Geometry check sheet. Reference: the model listing, model coordinates, mm. Face numbers are marked on the shaded views. Give positions to 0.01 mm unless a question says otherwise; leave off trailing zeros. Loops run counter-clockwise (first coordinate to the right, second up) from the corner with the lowest first, then second, coordinate; pieces in that order, holes last. Notation, with made-up numbers: (44, 46.25) -> (49, 46.25) arc R24 ccw to (49, 65.25) -> close; hole circle Ø11 at (5.25, 17.25). An arc over 180 degrees is marked (long way). Answer as a JSON object with one key per item and string values.
from build123d import *

# Parameters (mm, degrees)
CROQUIS1_W              = 60
CROQUIS1_H              = 116
CROQUIS1_R              = 1.5
SALIENTE_EXTRUIR1_DEPTH = 15
CROQUIS2_W              = 15
CROQUIS2_H              = 15
CORTAR_EXTRUIR1_DEPTH   = 132.457217375


with BuildPart() as part:
    # Croquis1 → Saliente-Extruir1 (new body)
    with BuildSketch(Plane(origin=(0, 0, 0), x_dir=(0, 0, -1), z_dir=(1, 0, 0))):
        with Locations((30, 58)):
            Rectangle(CROQUIS1_W, CROQUIS1_H)
        with Locations((54, 5)):
            Circle(CROQUIS1_R, mode=Mode.SUBTRACT)
        with Locations((36, 5)):
            Circle(CROQUIS1_R, mode=Mode.SUBTRACT)
        with Locations((36, 29)):
            Circle(CROQUIS1_R, mode=Mode.SUBTRACT)
        with Locations((54, 29)):
            Circle(CROQUIS1_R, mode=Mode.SUBTRACT)
        with Locations(Location((24, 29, 0), (0, 0, 180))):
            Circle(CROQUIS1_R, mode=Mode.SUBTRACT)
        with Locations(Location((24, 5, 0), (0, 0, 180))):
            Circle(CROQUIS1_R, mode=Mode.SUBTRACT)
        with Locations(Location((6, 5, 0), (0, 0, 180))):
            Circle(CROQUIS1_R, mode=Mode.SUBTRACT)
        with Locations(Location((6, 29, 0), (0, 0, 180))):
            Circle(CROQUIS1_R, mode=Mode.SUBTRACT)
        with Locations((6, 87)):
            Circle(CROQUIS1_R, mode=Mode.SUBTRACT)
        with Locations((6, 111)):
            Circle(CROQUIS1_R, mode=Mode.SUBTRACT)
        with Locations((24, 111)):
            Circle(CROQUIS1_R, mode=Mode.SUBTRACT)
        with Locations((24, 87)):
            Circle(CROQUIS1_R, mode=Mode.SUBTRACT)
        with Locations(Location((36, 87, 0), (0, 0, 180))):
            Circle(CROQUIS1_R, mode=Mode.SUBTRACT)
        with Locations(Location((36, 111, 0), (0, 0, 180))):
            Circle(CROQUIS1_R, mode=Mode.SUBTRACT)
        with Locations(Location((54, 111, 0), (0, 0, 180))):
            Circle(CROQUIS1_R, mode=Mode.SUBTRACT)
        with Locations(Location((54, 87, 0), (0, 0, 180))):
            Circle(CROQUIS1_R, mode=Mode.SUBTRACT)
        with Locations((32.5, 76.8)):
            Circle(CROQUIS1_R, mode=Mode.SUBTRACT)
        with Locations((32.5, 39.2)):
            Circle(CROQUIS1_R, mode=Mode.SUBTRACT)
    extrude(amount=SALIENTE_EXTRUIR1_DEPTH)

    # Croquis2 → Cortar-Extruir1 (cut, through all)
    with BuildSketch(Plane(origin=(15, 0, 0), x_dir=(0, 0, -1), z_dir=(1, 0, 0))):
        with Locations((7.5, 65.5)):
            Rectangle(CROQUIS2_W, CROQUIS2_H)
        with Locations((52.5, 50.5)):
            Rectangle(CROQUIS2_W, CROQUIS2_H)
    extrude(amount=-CORTAR_EXTRUIR1_DEPTH, mode=Mode.SUBTRACT)


solid = part.part
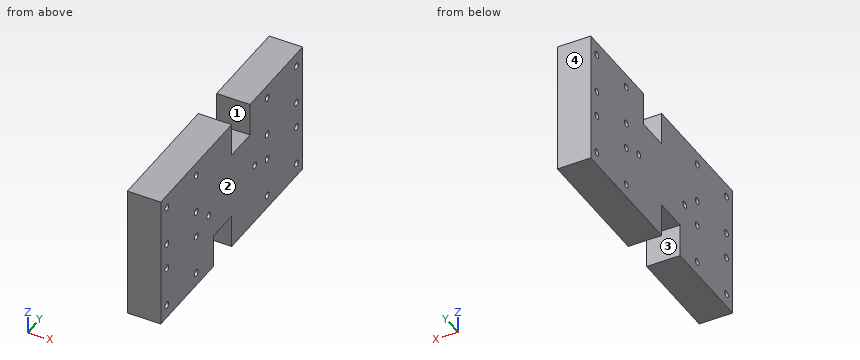
1) Section check A-A on z = -12. Record the cut outline in (x, y).
Geometry check:
{"outline": "(0, 0) -> (15, 0) -> (15, 58) -> (0, 58) -> close; (0, 73) -> (15, 73) -> (15, 116) -> (0, 116) -> close"}
2) Material ranges on line 1 along Z through (x, y) = (7.5, 111); line 2 along Y through (x, z) = (10, -36); line 3 along Y through (x, z) = (10.75, -6), recorded low to high. Write a range as from..to.
Geometry check:
{"line 1": "z = -60..-55.5, -52.5..-37.5, -34.5..-25.5, -22.5..-7.5, -4.5..0", "line 2": "y = 0..3.5, 6.5..27.5, 30.5..85.5, 88.5..109.5, 112.5..116", "line 3": "y = 0..3.5, 6.5..27.5, 30.5..58, 73..85.5, 88.5..109.5, 112.5..116"}
3) Section check D-D on x = 3. Count the separate pieces of the cut face and the enclosed holes in it, plus the area to 3 significant figures.
Geometry check:
{"separate pieces": "1", "enclosed holes": "18", "area": "6,380 mm2"}
4) Depth check by flat-ended pin: P1, Ø4, axis at y = 29, z = -24, coming from the +X side; P2, Ø7.5, axis at x = 6.5, y = 67.5, coming from the +Z side. Enter the tip coordinate at first touch or a pass-through.
Geometry check:
{"P1": "stops at x = 15", "P2": "stops at z = -15"}
5) Section check C-C on z = -24. Record the cut outline in (x, y).
Geometry check:
{"outline": "(0, 0) -> (15, 0) -> (15, 3.5) -> (0, 3.5) -> close; (0, 6.5) -> (15, 6.5) -> (15, 27.5) -> (0, 27.5) -> close; (0, 30.5) -> (15, 30.5) -> (15, 85.5) -> (0, 85.5) -> close; (0, 88.5) -> (15, 88.5) -> (15, 109.5) -> (0, 109.5) -> close; (0, 112.5) -> (15, 112.5) -> (15, 116) -> (0, 116) -> close"}
6) Draft check along Y on the marked faces 1, 2, 3 and 4. Enter one of: pulls with the +Y half, pulls with the -Y half, needs draft (parallel to the pull), parting line crosses it, or undercut.
Geometry check:
{"face 1": "undercut", "face 2": "needs draft", "face 3": "undercut", "face 4": "pulls with the +Y half"}
7) Section check B-B on y = 76.8. Record the cut outline in (x, z).
Geometry check:
{"outline": "(0, -60) -> (15, -60) -> (15, -34) -> (0, -34) -> close; (0, -31) -> (15, -31) -> (15, 0) -> (0, 0) -> close"}
